Work out the finished part from the listing and answer in its coordinate system (mm). Face numbers are marked on the shaded views. A direction names the side the tool comes from. Round coordinates to 2 decimals unless told otherwise and drop trailing zeros. Loops run counter-clockwise (first coordinate to the right, second up) from the corner with the lowest first, then second, coordinate; pieces in that order, holes last. Notation, with made-up numbers: (42, 56) -> (100, 56) arc R35 cw to (100, 90) -> close; hole circle Ø3 at (67.5, 10). An arc over 180 degrees is marked (long way). Use one line per item in the form item = value.
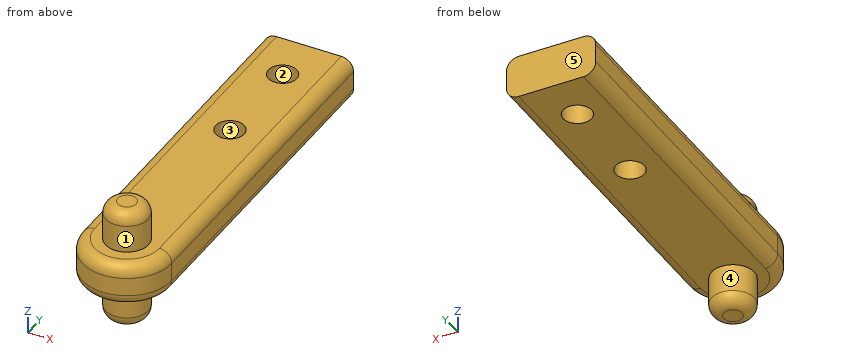
```python
from build123d import *

# Parameters (mm, degrees)
BOSS_EXTRUDE1_DEPTH          = 2.778125
BOSS_EXTRUDE1_DEPTH_BACK     = 2.778125
SKETCH2_R                    = 2.778125
BOSS_EXTRUDE2_DEPTH          = 7.9375
F_97_0_0059_DIAMETER_HOLE1_D = 3.699999966
FILLET1_R                    = 1.5875
FILLET2_R                    = 1.5875


with BuildPart() as part:
    # Sketch1 → Boss-Extrude1 (new, two sides: drawn at the far end of the back side and taken through both)
    with BuildSketch(Plane.XY.offset(-BOSS_EXTRUDE1_DEPTH_BACK)):
        with BuildLine():
            Line((20.579185749, 13.663463824), (20.579185749, 57.551094031))
            Line((20.579185749, 57.551094031), (9.003925336, 57.551094031))
            Line((9.003925336, 57.551094031), (9.003925336, 13.663463824))
            ThreePointArc((9.003925336, 13.663463824), (14.791555542, 7.875833618), (20.579185749, 13.663463824))
        make_face()
    extrude(amount=BOSS_EXTRUDE1_DEPTH + BOSS_EXTRUDE1_DEPTH_BACK)

    # Sketch2 → Boss-Extrude2 (add, symmetric)
    with BuildSketch(Plane.XY):
        with Locations(Location((14.791555542, 13.663463824, 0), (0, 0, 180))):
            Circle(SKETCH2_R)
    extrude(amount=BOSS_EXTRUDE2_DEPTH, both=True)

    # #97 (0.0059) Diameter Hole1 (through all)
    with Locations(Plane.XY.offset(2.778125)):
        with Locations((14.791555542, 51.201094031), (14.791555542, 38.501094031)):
            Hole(F_97_0_0059_DIAMETER_HOLE1_D / 2)

    # Fillet1
    fillet1_edges = [part.edges().sort_by_distance(p)[0] for p in [
        (17.569680542, 13.663463824, -7.9375),
        (17.569680542, 13.663463824, 7.9375),
    ]]
    fillet(fillet1_edges, radius=FILLET1_R)

    # Fillet2
    fillet2_edges = [part.edges().sort_by_distance(p)[0] for p in [
        (9.003925336, 35.607278928, 2.778125),
        (20.579185749, 35.607278928, 2.778125),
        (14.791555542, 7.875833618, 2.778125),
        (20.579185749, 35.607278928, -2.778125),
        (9.003925336, 35.607278928, -2.778125),
        (14.791555542, 7.875833618, -2.778125),
    ]]
    fillet(fillet2_edges, radius=FILLET2_R)


solid = part.part
```
(1) For the marked faces 1 and 2, determine the directions among +Z, -Z, +X, -X, +Y, -Y from which every point of the face is accessible in a straight line to the end or side of a thin tool.
Completed:
face_1 = +Z
face_2 = +Z, -Z
(2) Given P1, Ø4, axis at x = 13, y = 27, coming from the -Z side; P2, Ø3, axis at x = 14.79, y = 38.5, coming from the -Z side; P3, Ø8, axis at y = 13, z = -2.5, coming from the +X side; P4, Ø4, axis at x = 15, y = 29.5, coming from the +Z side, each flat-ended and moving along its own axis, determine where each tip first touches the part or whether it passes through.
Completed:
P1 = -2.78
P2 = through
P3 = 20.58
P4 = 2.78
(3) Find section B-B, the plane y = 22. Write down the section's boundary in (x, z) (1 decimal).
Completed:
outline = (9, -1.2) arc R1.6 ccw to (10.6, -2.8) -> (19, -2.8) arc R1.6 ccw to (20.6, -1.2) -> (20.6, 1.2) arc R1.6 ccw to (19, 2.8) -> (10.6, 2.8) arc R1.6 ccw to (9, 1.2) -> close
(4) Consider L1, parallel to Y at x = 15.75, z = -1; L2, parallel to Z at x = 11, y = 50; L3, parallel to X at y = 32.5, z = 2. Determine where each line is inside the solid, lowest interval first.
Completed:
L1 = 7.96 to 36.92, 40.08 to 49.62, 52.78 to 57.55
L2 = -2.78 to 2.78
L3 = 9.23 to 20.36
(5) Find section A-A, the plane y = 39.5. Write down the section's boundary in (x, z) (1 decimal), then the cut area to 3 significant figures.
Completed:
outline = (9, -1.2) arc R1.6 ccw to (10.6, -2.8) -> (13.2, -2.8) -> (13.2, 2.8) -> (10.6, 2.8) arc R1.6 ccw to (9, 1.2) -> close; (16.3, -2.8) -> (19, -2.8) arc R1.6 ccw to (20.6, -1.2) -> (20.6, 1.2) arc R1.6 ccw to (19, 2.8) -> (16.3, 2.8) -> close
area = 44.8 mm2
(6) Find section C-C, the plane z = 5.25. Write down the section's boundary in (x, y).
Completed:
outline = circle Ø5.56 at (14.79, 13.66)
(7) For a pull along Y with two mould halves and no side action, classify the marked faces 3, 4 and 5 as +Y half, -Y half, draft (parallel to the pull), parting line (faces both ways), or undercut.
Completed:
face_3 = undercut
face_4 = parting line
face_5 = +Y half
